Could you check a few things on this model? Use its own coordinates, in mm. A direction names the side the tool comes from. Give positions to 0.01 mm unless a question says otherwise; leave off trailing zeros. Write each loop counter-clockwise with the first axis right and the second up, starting at its lowest first coordinate (ties: lowest second). Pieces come first, ordered by that corner, then holes. Notation, with made-up numbers: (60.5, 2.5) -> (119.5, 2.5) arc R36 ccw to (119.5, 39.5) -> close; hole circle Ø6 at (0, 11.25). An arc over 180 degrees is marked (long way). Write item = value, one per line. Start each with the question number.
```python
from build123d import *

# Parameters (mm, degrees)
F0_W     = 36
F0_H     = 63
F1_DEPTH = 23
F2_SIZE  = 3
F4_DEPTH = 15


with BuildPart() as f1:
    # F0 (on Front) → F1 (new body)
    with BuildSketch(Plane.XZ):
        with BuildLine():
            ThreePointArc((36, 63), (18, 81), (0, 63))
            Line((0, 63), (36, 63))
        make_face()
        with Locations((18, 31.5)):
            Rectangle(F0_W, F0_H)
    extrude(amount=F1_DEPTH)

    # F2
    f2_edges = [f1.edges().sort_by_distance(p)[0] for p in [
        (18, -23, 81),
        (0, -23, 31.5),
        (18, -23, 0),
        (36, -23, 31.5),
    ]]
    chamfer(f2_edges, length=F2_SIZE)

    # F3 (on Front) → F4 (join)
    with BuildSketch(Plane.XZ):
        with BuildLine():
            ThreePointArc((8.550904, 78.320398), (9.400963, 78.813177), (10.276645, 79.258837))
            ThreePointArc((10.276645, 79.258837), (21.654333, 80.625148), (31.550904, 74.847911))
            Line((31.550904, 74.847911), (31.550904, 114.847911))
            Line((31.550904, 114.847911), (8.550904, 114.847911))
            Line((8.550904, 114.847911), (8.550904, 78.320398))
        make_face()
        with BuildLine():
            ThreePointArc((31.550904, 74.847911), (21.654333, 80.625148), (10.276645, 79.258837))
            ThreePointArc((10.276645, 79.258837), (9.400963, 78.813177), (8.550904, 78.320398))
            Line((8.550904, 78.320398), (8.550904, 74.847911))
            Line((8.550904, 74.847911), (31.550904, 74.847911))
        make_face()
    extrude(amount=F4_DEPTH)


solid = f1.part
```
(1) Imagine slicing it at A-A (x = 18). Please give me the cut outline in (y, z), then the cut area to 3 significant figures.
(2) On a 3-axis mill with a long thin cutter (end or side, diameter ignored), from which of +Z, -Z, +X, -X, +Y, -Y can I reach the whole of each face in a straight line? I mean faces 1 (the flat face through (31.551, -7, 95)), 2 (the flat face through (18, -22, 2)), 3 (the flat face through (8.551, -7, 97)). Say none if no direction works.
(3) If I drill on line 1 along X through (y, z) = (-13, 89); line 2 along Y through (x, z) = (11, 82); line 3 along Y through (x, z) = (2, 8.5), over which ranges is the centre line in solid material (lowest first)? Write a range as from..to.
(4) Imagine slicing it at D-D (y = -18.75). Please give me the cut outline in (x, z).
(5) Imagine slicing it at C-C (z = 87). Please give me the cut outline in (x, y), then the cut area to 3 significant figures.
(6) I'm going to push flat-ended pins straight in: pin 1 (12 mm diameter, centred on x = 28.5, z = 85.5, fed in from -Y); pin 2 (8 mm diameter, centred on y = -20, z = 81.5, fed in from +X); pin 3 (7.5 mm diameter, centred on y = -8.5, z = 101, fed in from +X). Where does each tip first touch, or does it pass through?
(7) Imagine slicing it at B-B (y = -5.5). Please give me the cut outline in (x, z), then the cut area to 3 significant figures.
Answers below:
q1.outline = (-23, 3) -> (-20, 0) -> (0, 0) -> (0, 114.85) -> (-15, 114.85) -> (-15, 81) -> (-20, 81) -> (-23, 78) -> close
q1.area = 2,360 mm^2
q2.face_1 = +Z, +X, +Y, -Y
q2.face_2 = -Z, +X, -X, -Y
q2.face_3 = +Z, -X, +Y, -Y
q3.line_1 = 8.55..31.55
q3.line_2 = -15..0
q3.line_3 = -22..0
q4.outline = (0, 0) -> (36, 0) -> (36, 63) arc R18 ccw to (0, 63) -> close
q5.outline = (8.55, -15) -> (31.55, -15) -> (31.55, 0) -> (8.55, 0) -> close
q5.area = 345 mm^2
q6.pin_1 = -15
q6.pin_2 = 28.67
q6.pin_3 = 31.55
q7.outline = (0, 0) -> (36, 0) -> (36, 63) arc R18 ccw to (31.55, 74.85) -> (31.55, 114.85) -> (8.55, 114.85) -> (8.55, 78.32) arc R18 ccw to (0, 63) -> close
q7.area = 3,590 mm^2
